Read the model definition and answer for the solid it produces. Units are mm, in the model's axes. A direction names the side the tool comes from. Round coordinates to 2 decimals unless told otherwise and drop trailing zeros. Write each loop counter-clockwise with the first axis right and the second up, starting at its lowest first coordinate (ties: lowest second). Pieces come first, ordered by that corner, then holes. Notation, with made-up numbers: (50, 40.25) -> (57, 40.25) arc R29 cw to (57, 67.25) -> close; hole circle Ø1 at (36, 78). An arc over 180 degrees is marked (long way). Return JSON: item names as keys, results as strings. Group by question number.
(1) A cutting plane is placed at C-C on y = 6. Give the vertices of the cut face in (x, z).
(2) A cutting plane is placed at B-B on x = -7. Give the vertices of the cut face in (y, z), then the cut area to 3 significant figures.
(3) A cutting plane is placed at A-A on z = 0.75. Give the vertices of the cut face in (x, y).
(4) The mould has two halves that part along Z. Classify faces 1 (the flat face through (-10, 11, 0)), 2 (the flat face through (0, 11, 2)), 3 (the cylindrical face through (-10.07, 28.39, 12.1)): released by +Z, released by -Z, zero draft, split by the parting line, or undercut.
(5) For faces 4 (the flat face through (-3.244, 26.586, 6.451)), 5 (the flat face through (-16.706, 26.66, 6.451)), 6 (the flat face through (-10, 11, -4)), 7 (the flat face through (-8, 24, 6)), determine the directions among +Z, -Z, +X, -X, +Y, -Y from which every point of the face is accessible in a straight line to the end or side of a thin tool.
(6) A cutting plane is placed at D-D on z = 8. Give the vertices of the cut face in (x, y), then the cut area to 3 significant figures.
(7) Given pin 1 (10 mm diameter, centred on x = -15, y = 9.5, fed in from +Z); pin 2 (1.4 mm diameter, centred on x = -7, y = 4, fed in from +Z); pin 3 (2 mm diameter, centred on y = 25, z = -4, fed in from +X); pin 4 (8 mm diameter, centred on x = -8.5, z = 9.5, fed in from -Y), each flat-ended and moving along its own axis, determine where each tip first touches the part or whether it passes through.
(8) Straight lines are drawn through the part: line 1 (X direction, y = 4, z = -5.05); line 2 (Y direction, x = -13, z = 1.1); line 3 (Z direction, x = -5.25, y = 6.5). For each, find the intervals that lie inside material, in ascending order.
```python
from build123d import *

# Parameters (mm, degrees)
SKETCH_R        = 1.2
PAD_DEPTH       = 3
PAD001_DEPTH    = 10
FILLET_R        = 3
SKETCH002_R     = 2.5
POCKET_DEPTH    = 6
SKETCH003_R     = 1.2
PAD002_DEPTH    = 7
SKETCH004_W     = 20
SKETCH004_H     = 4
POCKET001_DEPTH = 22


with BuildPart() as part:
    # Sketch → Pad (new body)
    with BuildSketch(Plane.XY):
        Polygon((-20, 22), (-20, 0), (0, 0), (0, 22), (-5, 29.412805), (-15, 29.412805), align=None)
        with Locations((-7, 4)):
            Circle(SKETCH_R, mode=Mode.SUBTRACT)
        with Locations((-13, 4)):
            Circle(SKETCH_R, mode=Mode.SUBTRACT)
    extrude(amount=PAD_DEPTH)

    # Sketch001 (on Face10 of Pad) → Pad001 (join)
    with BuildSketch(Plane.XY.offset(3)):
        Polygon((-10, 24), (-1.5, 24), (-5.038419, 29.245922), (-14.961581, 29.245922), (-18.5, 24), align=None)
    extrude(amount=PAD001_DEPTH)

    # Fillet
    fillet_edges = [part.edges().sort_by_distance(p)[0] for p in [
        (-3.26921, 26.622961, 13),
        (-10, 29.245922, 13),
        (-16.73079, 26.622961, 13),
    ]]
    fillet(fillet_edges, radius=FILLET_R)

    # Sketch002 (on Face1 of Fillet) → Pocket (cut)
    with BuildSketch(Plane.XZ.offset(-24)):
        with Locations((-10, 8)):
            Circle(SKETCH002_R)
    extrude(amount=-POCKET_DEPTH, mode=Mode.SUBTRACT)

    # Sketch003 (on Face20 of Pocket) → Pad002 (join)
    with BuildSketch(Plane(origin=(0, 0, 0), x_dir=(1, 0, 0), z_dir=(0, 0, -1))):
        Polygon((0, 0), (-20, 0), (-20, -22), (-15, -29.412805), (-5, -29.412805), (0, -22), align=None)
        with Locations((-13, -4)):
            Circle(SKETCH003_R, mode=Mode.SUBTRACT)
        with Locations((-7, -4)):
            Circle(SKETCH003_R, mode=Mode.SUBTRACT)
    extrude(amount=PAD002_DEPTH)

    # Sketch004 (on Face22 of Pad002) → Pocket001 (cut)
    with BuildSketch(Plane.XZ):
        with Locations((-10, -2)):
            Rectangle(SKETCH004_W, SKETCH004_H)
    extrude(amount=-POCKET001_DEPTH, mode=Mode.SUBTRACT)


solid = part.part
```
Checks:
{
 "1": {"outline": "(-20, -7) -> (0, -7) -> (0, -4) -> (-20, -4) -> close; (-20, 0) -> (0, 0) -> (0, 3) -> (-20, 3) -> close"},
 "2": {"outline": "(0, -7) -> (2.8, -7) -> (2.8, -4) -> (0, -4) -> close; (0, 0) -> (2.8, 0) -> (2.8, 3) -> (0, 3) -> close; (5.2, -7) -> (29.41, -7) -> (29.41, 3) -> (29.25, 3) -> (29.25, 10) arc R3 ccw to (26.25, 13) -> (24, 13) -> (24, 3) -> (5.2, 3) -> (5.2, 0) -> (22, 0) -> (22, -4) -> (5.2, -4) -> close", "area": "242 mm^2"},
 "3": {"outline": "(-20, 0) -> (0, 0) -> (0, 22) -> (-5, 29.41) -> (-15, 29.41) -> (-20, 22) -> close; hole circle Ø2.4 at (-13, 4); hole circle Ø2.4 at (-7, 4)"},
 "4": {"face 1": "undercut", "face 2": "zero draft", "face 3": "released by +Z"},
 "5": {"face 4": "+Z, +X, +Y", "face 5": "+Z, -X, +Y", "face 6": "+X, -X, -Y", "face 7": "+Z, +X, -X, -Y"},
 "6": {"outline": "(-18.5, 24) -> (-12.5, 24) -> (-12.5, 29.25) -> (-14.96, 29.25) -> close; (-7.5, 24) -> (-1.5, 24) -> (-5.04, 29.25) -> (-7.5, 29.25) -> close", "area": "44.4 mm^2"},
 "7": {"pin 1": "stops at z = 3", "pin 2": "passes through", "pin 3": "stops at x = -1.35", "pin 4": "stops at y = 24"},
 "8": {"line 1": "x = -20 to -14.2, -11.8 to -8.2, -5.8 to 0", "line 2": "y = 0 to 2.8, 5.2 to 29.41", "line 3": "z = -7 to -4, 0 to 3"}
}
